Read the model definition and answer for the solid it produces. Units are mm, in the model's axes. Coordinates: 2 decimals unless noted, no trailing zeros. Order: outer loops, then holes, each group sorted by start corner. A loop starts at its lowest first (then second) coordinate and runs counter-clockwise, first axis right, second up. Notation, with made-up numbers: M -16,-20 L 9,-20 A32 ccw 9,10 Z; hole C 83.5,86 d8. An arc over 180 degrees is marked long. Use a Markdown table: item, result. Add a question column.
1) The mould has two halves that part along X. Classify faces 1 (the face through (-4.68, 4.29, 2.95)), 2 (the face through (2.93, -5.634, 18.808)), 3 (the face through (-1, 7, 25.4)), 4 (the face through (-9.516, 0.419, 12.529)): released by +X, released by -X, zero draft, split by the parting line, or undercut.
2) Find section C-C on z = 17.5. Write down the section's boundary in (x, y) (3 decimals), plus the area to 3 significant figures.
3) Find section A-A on x = 0. Write down the section's boundary in (y, z) (3 decimals).
4) Find section B-B on z = 11.75. Write down the section's boundary in (x, y) (3 decimals).
5) Find the intervals of material crossed by probe 1 along Y at (x, z) = (0, 16.25) (3 decimals); probe 2 along Z at (x, y) = (0, 7) (3 decimals); probe 3 along X at (y, z) = (6.75, 6), in increasing order. Write a range as [from, to].
6) Find section D-D on x = -6. Count the separate pieces of the cut face and the enclosed holes in it, plus the area to 3 significant figures.
7) Each of these flat-tipped pins is pushed along its axis until it touches: pin 1 Ø1 at (x, y) = (-7.5, -6.5) entering from +Z; pin 2 Ø3 at (x, z) = (4.5, 18) entering from +Y; pin 3 Ø3 at (x, z) = (-7, 5) entering from +Y; pin 4 Ø10 at (x, z) = (0.5, 19) entering from +Y (3 decimals). Where does it stop, or does it pass through?
from build123d import *

# Parameters (mm, degrees)
F0_R     = 9.525
F0_R_2   = 6.35
F1_DEPTH = 25.4
F3_DEPTH = 12.7
F4_SIZE  = 0.508


with BuildPart() as f1:
    # F0 (on Top) → F1 (new body)
    with BuildSketch(Plane.XY):
        Circle(F0_R)
        Circle(F0_R_2, mode=Mode.SUBTRACT)
    extrude(amount=F1_DEPTH)

    # F2 (on Front) → F3 (cut, symmetric)
    with BuildSketch(Plane.XZ):
        with BuildLine():
            ThreePointArc((-6.35, 9.525), (0, 3.175), (6.35, 9.525))
            ThreePointArc((6.35, 9.525), (0, 15.875), (-6.35, 9.525))
        make_face()
    extrude(amount=F3_DEPTH, both=True, mode=Mode.SUBTRACT)

    # F4
    f4_edges = [f1.edges().sort_by_distance(p)[0] for p in [
        (-6.35, 0, 25.4),
        (-9.525, 0, 25.4),
        (-6.35, 0, 0),
        (-9.525, 0, 0),
    ]]
    chamfer(f4_edges, length=F4_SIZE)


solid = f1.part
Check result:
| question | item | result |
|---|---|---|
| 1 | face 1 | undercut |
| 1 | face 2 | undercut |
| 1 | face 3 | zero draft |
| 1 | face 4 | split by the parting line |
| 2 | outline | C 0,0 d19.05; hole C 0,0 d12.7 |
| 2 | area | 158 mm2 |
| 3 | outline | M -9.525,0.508 L -9.017,0 L -6.858,0 L -6.35,0.508 L -6.35,3.175 L -9.525,3.175 Z; M -9.525,15.875 L -6.35,15.875 L -6.35,24.892 L -6.858,25.4 L -9.017,25.4 L -9.525,24.892 Z; M 6.35,0.508 L 6.858,0 L 9.017,0 L 9.525,0.508 L 9.525,3.175 L 6.35,3.175 Z; M 6.35,15.875 L 9.525,15.875 L 9.525,24.892 L 9.017,25.4 L 6.858,25.4 L 6.35,24.892 Z |
| 4 | outline | M -5.947,-7.44 L -5.947,-2.225 A6.35 cw -5.947,2.225 L -5.947,7.44 A9.525 ccw Z; M 5.947,-7.44 A9.525 ccw 5.947,7.44 L 5.947,2.225 A6.35 cw 5.947,-2.225 Z |
| 5 | probe 1 | y = [-9.525, -6.35], [6.35, 9.525] |
| 5 | probe 2 | z = [0, 3.175], [15.875, 25.4] |
| 5 | probe 3 | x = [-6.72, -5.28], [5.28, 6.72] |
| 6 | separate pieces | 4 |
| 6 | enclosed holes | 0 |
| 6 | area | 224 mm2 |
| 7 | pin 1 | stops at z = 24.99 |
| 7 | pin 2 | stops at y = 9.04 |
| 7 | pin 3 | stops at y = 7.78 |
| 7 | pin 4 | stops at y = 9.525 |
